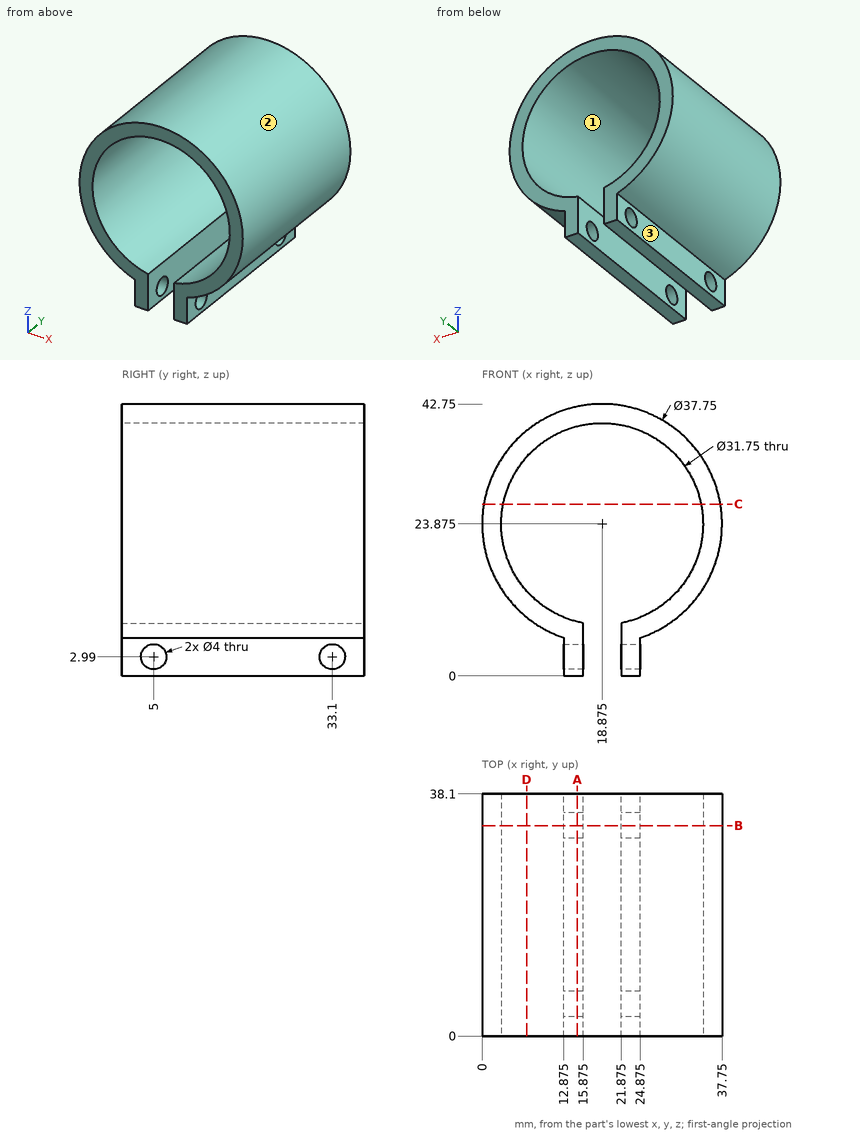
Geometry check sheet. Reference: drawing and pictorial views, mm from the part's lowest x, y, z. Coordinates: 2 decimals unless noted, no trailing zeros. Order: outer loops, then holes, each group sorted by start corner. A loop starts at its lowest first (then second) coordinate and runs counter-clockwise, first axis right, second up. Notation, with made-up numbers: (47.25, 7.25) -> (93.25, 7.25) arc R8 ccw to (93.25, 13.25) -> close; hole circle Ø4 at (49.25, -9). An arc over 180 degrees is marked (long way). Put each result on its own line as item: value. Start each with the question number.
1) Cross-section at C-C (z = 27). Enter the section's corners in (x, y).
2) Cross-section at A-A (x = 15). Enter the section's corners in (y, z), plus the area to 3 significant figures.
3) Cross-section at D-D (x = 7). Enter the section's corners in (y, z), plus the area to 3 significant figures.
4) Go/stop test with flat-tipped pins: pin 1 (9 mm diameter, centred on y = 22, z = 3.5, fed in from -X) (1 decimal); pin 2 (12 mm diameter, centred on x = 33.5, y = 8, fed in from +Z) (1 decimal); pin 3 (3 mm diameter, centred on y = 9.5, z = 4, fed in from +X) (1 decimal); pin 4 (12 mm diameter, centred on y = 33.5, z = 30, fed in from +X). Record where each tip stops, or that it passes through.
5) Release check for a two-part mould opening along Z. For the marked faces 1, 2 and 3 record: pulls with the +Z half, pulls with the -Z half, needs draft (parallel to the pull), parting line crosses it, or undercut.
6) Cross-section at B-B (y = 33.1). State how many separate pieces and enclosed holes the cut face has, plus the area to 3 significant figures.
7) Material ranges on L1, parallel to X at y = 7.5, z = 24; L2, parallel to Z at x = 27, y = 19.5 (1 decimal); L3, parallel to X at y = 29.5, z = 10 (1 decimal), recorded low to high.
Geometry check:
1. outline: (0.26, 0) -> (3.31, 0) -> (3.31, 38.1) -> (0.26, 38.1) -> close; (34.44, 0) -> (37.49, 0) -> (37.49, 38.1) -> (34.44, 38.1) -> close
2. outline: (0, 0) -> (38.1, 0) -> (38.1, 8.48) -> (0, 8.48) -> close; (0, 39.27) -> (38.1, 39.27) -> (38.1, 42.35) -> (0, 42.35) -> close; hole circle Ø4 at (5, 2.99); hole circle Ø4 at (33.1, 2.99)
2. area: 415 mm^2
3. outline: (0, 9.2) -> (38.1, 9.2) -> (38.1, 13.34) -> (0, 13.34) -> close; (0, 34.41) -> (38.1, 34.41) -> (38.1, 38.55) -> (0, 38.55) -> close
3. area: 315 mm^2
4. pin 1: stops at x = 8.7
4. pin 2: stops at z = 40.7
4. pin 3: stops at x = 24.9
4. pin 4: stops at x = 37.75
5. face 1: undercut
5. face 2: parting line crosses it
5. face 3: needs draft
6. separate pieces: 3
6. enclosed holes: 0
6. area: 319 mm^2
7. L1: x = 0 to 3, 34.75 to 37.75
7. L2: z = 6.8 to 10.2, 37.5 to 40.9
7. L3: x = 6.1 to 11.2, 26.6 to 31.7
